```python
from build123d import *

# Parameters (mm, degrees)
SKETCH1_R           = 50.8
BOSS_EXTRUDE1_DEPTH = 50
SKETCH4_R           = 4
SKETCH4_R_2         = 2
CUT_EXTRUDE2_DEPTH  = 71


with BuildPart() as part:
    # Sketch1 → Boss-Extrude1 (new body)
    with BuildSketch(Plane(origin=(0, 0, 0), x_dir=(1, 0, 0), z_dir=(0, 1, 0))):
        Circle(SKETCH1_R)
    extrude(amount=BOSS_EXTRUDE1_DEPTH)

    # Sketch3 → Cut-Revolve1 (revolve, cut)
    with BuildSketch(Plane.XY):
        Polygon((0, 0), (38.1, 0), (38.1, 2), (36.5, 2), (0, 38.5), align=None)
    revolve(axis=Axis((0, 38.5, 0), (0, -1, 0)), mode=Mode.SUBTRACT)

    # Sketch4 → Cut-Extrude2 (cut)
    with BuildSketch(Plane(origin=(0, 50, 0), x_dir=(1, 0, 0), z_dir=(0, 1, 0))):
        Circle(SKETCH4_R)
        with Locations((0, 44.8)):
            Circle(SKETCH4_R_2)
        with Locations((38.79793809, 22.4)):
            Circle(SKETCH4_R_2)
        with Locations((38.79793809, -22.4)):
            Circle(SKETCH4_R_2)
        with Locations((0, -44.8)):
            Circle(SKETCH4_R_2)
        with Locations((-38.79793809, -22.4)):
            Circle(SKETCH4_R_2)
        with Locations((-38.79793809, 22.4)):
            Circle(SKETCH4_R_2)
    extrude(amount=-CUT_EXTRUDE2_DEPTH, mode=Mode.SUBTRACT)


solid = part.part
```
Verification items for the finished model (mm, model axes). A direction names the side the tool comes from. Give positions to 0.01 mm unless a question says otherwise; leave off trailing zeros. Order: outer loops, then holes, each group sorted by start corner. A loop starts at its lowest first (then second) coordinate and runs counter-clockwise, first axis right, second up. Notation, with made-up numbers: M -4.5,64.25 L 54.5,64.25 A29 ccw 54.5,89.25 Z; hole C -14,-13 d7. An arc over 180 degrees is marked long. Answer in a Markdown table with one row per item. Add a question column.
Item 1: Section check A-A, the plane y = 27. Enter the section's corners in (x, z), and give its area (3 significant figures).
Item 2: Tool access check on faces 4 (the cylindrical face through (-30.235, 1.014, -23.183)), 5 (the cylindrical face through (36.8, 25.4, 22.3)). Record the directions out of +Z, -Z, +X, -X, +Y, -Y that give a thin tool (end or side, any length) a straight path to the whole face; none if there is none.
Item 3: Scan lines: probe 1 along Z at (x, y) = (0, 40); probe 2 along Z at (x, y) = (0, 26.5); probe 3 along X at (y, z) = (40, 22.4). Record each from-to range of solid material in increasing order. Write a range as from..to.
Item 4: Section check D-D, the plane y = 41. Enter the section's corners in (x, z).
Item 5: Gauge pin test, flat ends, axial feed: pin 1 (5 mm diameter, centred on x = -1, z = 35.5, fed in from -Y); pin 2 (3 mm diameter, centred on x = 0, z = 44.8, fed in from -Y); pin 3 (3 mm diameter, centred on x = 21.5, z = -16, fed in from -Y); pin 4 (3 mm diameter, centred on y = 29, z = 12.5, fed in from -X). Record the tip position at first contact, or that the pin passes through.
Item 6: Section check C-C, the plane z = -44.8. Enter the section's corners in (x, y), and give its area (4 significant figures).
Item 7: Section check B-B, the plane x = 0. Enter the section's corners in (y, z).
Item 8: Mould release check, pull along X, two halves, no side actions. Record for faces 1 (the flat face through (-8, 0, -38)), 2 (the cylindrical face through (-0.26, 25.35, -46.783)), 3 (the cylindrical face through (-11.012, 24.65, 49.592)): released by +X, released by -X, zero draft, split by the parting line, or undercut.
Filled sheet:
| question | item | result |
|---|---|---|
| 1 | outline | C 0,0 d101.6; hole C -38.8,-22.4 d4; hole C -38.8,22.4 d4; hole C 0,0 d23; hole C 0,-44.8 d4; hole C 0,44.8 d4; hole C 38.8,-22.4 d4; hole C 38.8,22.4 d4 |
| 1 | area | 7,620 mm^2 |
| 2 | face 4 | -Y |
| 2 | face 5 | +Y, -Y |
| 3 | probe 1 | z = -50.8..-46.8, -42.8..-4, 4..42.8, 46.8..50.8 |
| 3 | probe 2 | z = -50.8..-46.8, -42.8..-12, 12..42.8, 46.8..50.8 |
| 3 | probe 3 | x = -45.59..-40.8, -36.8..36.8, 40.8..45.59 |
| 4 | outline | C 0,0 d101.6; hole C -38.8,-22.4 d4; hole C -38.8,22.4 d4; hole C 0,0 d8; hole C 0,-44.8 d4; hole C 0,44.8 d4; hole C 38.8,-22.4 d4; hole C 38.8,22.4 d4 |
| 5 | pin 1 | stops at y = 2 |
| 5 | pin 2 | passes through |
| 5 | pin 3 | stops at y = 10.2 |
| 5 | pin 4 | stops at x = -49.59 |
| 6 | outline | M -23.95,0 L -2,0 L -2,50 L -23.95,50 Z; M 2,0 L 23.95,0 L 23.95,50 L 2,50 Z |
| 6 | area | 2,195 mm^2 |
| 7 | outline | M 0,-50.8 L 50,-50.8 L 50,-46.8 L 0,-46.8 Z; M 0,-42.8 L 50,-42.8 L 50,-4 L 34.5,-4 L 2,-36.5 L 2,-38.1 L 0,-38.1 Z; M 0,38.1 L 2,38.1 L 2,36.5 L 34.5,4 L 50,4 L 50,42.8 L 0,42.8 Z; M 0,46.8 L 50,46.8 L 50,50.8 L 0,50.8 Z |
| 8 | face 1 | zero draft |
| 8 | face 2 | undercut |
| 8 | face 3 | split by the parting line |
